Read the model definition and answer for the solid it produces. Units are mm, in the model's axes. A direction names the side the tool comes from. Coordinates: 2 decimals unless noted, no trailing zeros. Write each loop counter-clockwise with the first axis right and the second up, starting at its lowest first coordinate (ties: lowest second). Pieces come first, ordered by that corner, then holes. Notation, with made-up numbers: (88.5, -29) - (128.5, -29) arc R21 ccw to (128.5, -24) - close; hole circle Ø7 at (73, -23). An arc over 180 degrees is marked (long way). Use a Markdown table: item, result.
Autodesk Inventor part; units mm, degrees
ref_plane "Arbeitsebene1" through (0, 0, 0) normal (-1, 0, 0) x (0, -1, 0)
ref_plane "Arbeitsebene7" through (0, 0, 2.2393) normal (0, 0, 1) x (1, 0, 0)
ref_plane "Arbeitsebene10" through (0, 0, 32.2393) normal (-1, 0, 0) x (0, 0, 1)
ref_plane "Arbeitsebene1" through (0, 0, 0) normal (-1, 0, 0) x (0, -1, 0)
ref_plane "Arbeitsebene7" through (0, 0, 2.2393) normal (0, 0, 1) x (1, 0, 0)
sketch "Skizze6" plane through (0, 0, 2.2393) normal (0, 0, 1) x (1, 0, 0)
  circle A0 centre (0, 0) radius 1.1115
extrude "Extrusion6" add sketch "Skizze6" along normal blind 30
ref_plane "Arbeitsebene10" through (0, 0, 32.2393) normal (-1, 0, 0) x (0, 0, 1)
sketch "Skizze8" plane through (0, 0, 32.2393) normal (-1, 0, 0) x (0, 0, 1)
  line L0 (0, 0) -> (3, 0)
  line L1 (0, 0) -> (0, 2)
  line L2 (0, 2) -> (3, 0)
  line L3 (-42.2872, 0) -> (10.5479, 0)
  point P0 (-32.2393, 0)
  dimension "d17" = 3
  dimension "d18" = 2
revolve "Umdrehung2" add sketch "Skizze8" angle 360 about axis through (0, 0, 32.2393) along (0, 0, 1)
sketch "Skizze11" plane through (0, 0, 2.2393) normal (0, 0, -1) x (-1, 0, 0)
  circle A0 centre (0, 0) radius 0.5
  dimension "d26" = 1
extrude "Extrusion7" add sketch "Skizze11" along normal blind 1.5
properties part number "xyz_Axis_with_ball_Axis"
(1) For faces 1 (the flat face through (0, 0, 0.739)), 2 (the flat face through (1, 1, 32.239)), determine the directions among +Z, -Z, +X, -X, +Y, -Y from which every point of the face is accessible in a straight line to the end or side of a thin tool.
Report:
| item | result |
|---|---|
| face 1 | -Z, +X, -X, +Y, -Y |
| face 2 | -Z |
(2) A cutting plane is placed at B-B, the plane z = 33. Write down the section's boundary in (x, y), and give its area (3 significant figures).
Report:
| item | result |
|---|---|
| outline | circle Ø2.99 at (0, 0) |
| area | 7.00 mm² |
(3) Straight lines are drawn through the part: L1, parallel to X at y = -0.1, z = 4; L2, parallel to Z at x = -0.6, y = 0.9; L3, parallel to X at y = 0.8, z = 21. For each, find the intervals that lie inside material, in ascending order.
Report:
| item | result |
|---|---|
| L1 | x = -1.11 to 1.11 |
| L2 | z = 2.24 to 33.62 |
| L3 | x = -0.77 to 0.77 |
(4) Each of these flat-tipped pins is pushed along its axis until it touches: P1, Ø1, axis at x = 0, z = 30, coming from the -Y side; P2, Ø2, axis at x = 1, y = 0, coming from the -Z side. Where does it stop, or does it pass through?
Report:
| item | result |
|---|---|
| P1 | stops at y = -1.11 |
| P2 | stops at z = 0.74 |
(5) A cutting plane is placed at A-A, the plane z = 3.5. Write down the section's boundary in (x, y), and give its area (3 significant figures).
Report:
| item | result |
|---|---|
| outline | circle Ø2.22 at (0, 0) |
| area | 3.88 mm² |
